```python
from build123d import *

# Parameters (mm, degrees)
F0_R     = 132.5
F0_R_2   = 9.5
F1_DEPTH = 18
F2_R     = 2
F3_R     = 132.5
F3_R_2   = 9.5
F3_R_3   = 103
F4_DEPTH = 2
F5_R     = 1.99999
F6_R     = 77.5
F7_DEPTH = 18.001
F6_R_2   = 92.6
F8_DEPTH = 11
F9_SIZE  = 3


# Not quite as in the source:
# - a fillet or chamfer is up to 0.001 mm smaller than in the source, because OpenCascade refuses the exact size


with BuildPart() as f1:
    # F0 (on Front) → F1 (new body)
    with BuildSketch(Plane.XZ):
        Circle(F0_R)
        with Locations((-44.008594722, -106.2461462388)):
            Circle(F0_R_2, mode=Mode.SUBTRACT)
        with Locations((-106.2461462388, -44.008594722)):
            Circle(F0_R_2, mode=Mode.SUBTRACT)
        with Locations((44.008594722, -106.2461462388)):
            Circle(F0_R_2, mode=Mode.SUBTRACT)
        with Locations((106.2461462388, -44.008594722)):
            Circle(F0_R_2, mode=Mode.SUBTRACT)
        with Locations((-106.2461462388, 44.008594722)):
            Circle(F0_R_2, mode=Mode.SUBTRACT)
        with Locations((-44.008594722, 106.2461462388)):
            Circle(F0_R_2, mode=Mode.SUBTRACT)
        with Locations((106.2461462388, 44.008594722)):
            Circle(F0_R_2, mode=Mode.SUBTRACT)
        with Locations((44.008594722, 106.2461462388)):
            Circle(F0_R_2, mode=Mode.SUBTRACT)
    extrude(amount=F1_DEPTH)

    # F2
    f2_edges = [f1.edges().sort_by_distance(p)[0] for p in [
        (-132.5, -18, 0),
    ]]
    fillet(f2_edges, radius=F2_R)

    # F3 (on face) → F4 (cut)
    with BuildSketch(Plane(origin=(0, 0, 0), x_dir=(-1, 0, 0), z_dir=(0, 1, 0))):
        Circle(F3_R)
        with Locations((-44.008594722, -106.2461462388)):
            Circle(F3_R_2, mode=Mode.SUBTRACT)
        with Locations((-106.2461462388, -44.008594722)):
            Circle(F3_R_2, mode=Mode.SUBTRACT)
        with Locations((44.008594722, -106.2461462388)):
            Circle(F3_R_2, mode=Mode.SUBTRACT)
        with Locations((106.2461462388, -44.008594722)):
            Circle(F3_R_2, mode=Mode.SUBTRACT)
        with Locations((-106.2461462388, 44.008594722)):
            Circle(F3_R_2, mode=Mode.SUBTRACT)
        with Locations((-44.008594722, 106.2461462388)):
            Circle(F3_R_2, mode=Mode.SUBTRACT)
        Circle(F3_R_3, mode=Mode.SUBTRACT)
        with Locations((106.2461462388, 44.008594722)):
            Circle(F3_R_2, mode=Mode.SUBTRACT)
        with Locations((44.008594722, 106.2461462388)):
            Circle(F3_R_2, mode=Mode.SUBTRACT)
    extrude(amount=-F4_DEPTH, mode=Mode.SUBTRACT)

    # F5 (radius 2 in the source; OpenCascade refuses exactly that, so slightly less here)
    f5_edges = [f1.edges().sort_by_distance(p)[0] for p in [
        (103, -2, 0),
    ]]
    fillet(f5_edges, radius=F5_R)

    # F6 (on face) → F7 (cut, through all)
    with BuildSketch(Plane(origin=(0, 0, 0), x_dir=(-1, 0, 0), z_dir=(0, 1, 0))):
        Circle(F6_R)
    extrude(amount=-F7_DEPTH, mode=Mode.SUBTRACT)

    # F6 (on face) → F8 (cut)
    with BuildSketch(Plane(origin=(0, 0, 0), x_dir=(-1, 0, 0), z_dir=(0, 1, 0))):
        Circle(F6_R_2)
        Circle(F6_R, mode=Mode.SUBTRACT)
    extrude(amount=-F8_DEPTH, mode=Mode.SUBTRACT)

    # F9
    f9_edges = [f1.edges().sort_by_distance(p)[0] for p in [
        (77.5, -18, 0),
    ]]
    chamfer(f9_edges, length=F9_SIZE)


solid = f1.part
```
Can you work these out from the model? Positions are in its coordinate system, mm. A direction names the side the tool comes from. Coordinates: 2 decimals unless noted, no trailing zeros. Return JSON: item names as keys, results as strings.
Q1. Please list where these lines run through material, in increasing order: L1, parallel to Z at x = 0, y = -13; L2, parallel to X at y = -13.75, z = 102.5; L3, parallel to Z at x = -113, y = -15.25. Write a range as from..to.
Computed values:
{"L1": "z = -132.5..-77.5, 77.5..132.5", "L2": "x = -83.96..-52.74, -35.28..35.28, 52.74..83.96", "L3": "z = -69.19..-50.69, -37.33..37.33, 50.69..69.19"}
Q2. If we section it at C-C (y = -7.75): Count the separate pieces of the cut face and the enclosed holes in it, then the cut area to 3 significant figures.
Computed values:
{"separate pieces": "1", "enclosed holes": "9", "area": "25,900 mm2"}
Q3. Thinking about a two-plate mould opening in X: for faces 1 (the cylindrical face through (-34.95, -9.89, -103.39)), 2 (the cylindrical face through (71.231, -8.902, 111.725)), 3 (the flat face through (10, -2, -107)), which applies, +X half, -X half, draft (parallel to the pull), parting line (faces both ways), or undercut?
Computed values:
{"face 1": "undercut", "face 2": "parting line", "face 3": "draft"}
Q4. On a 3-axis mill with a long thin cutter (end or side, diameter ignored), from which of +Z, -Z, +X, -X, +Y, -Y can I reach the whole of each face in a straight line? I mean faces 4 (the cylindrical face through (92.51, -5.42, 4.07)), 5 (the cylindrical face through (16.8, -12.972, -75.657)). Say none if no direction works.
Computed values:
{"face 4": "+Y", "face 5": "+Y, -Y"}
Q5. I'm going to push flat-ended pins straight in: pin 1 Ø4 at (x, y) = (-17, -12.5) entering from -Z; pin 2 Ø22 at (x, z) = (-44.01, 106.25) entering from +Y; pin 3 Ø10 at (y, z) = (-10.5, -62) entering from -X; pin 4 Ø24.5 at (x, z) = (106.25, -44.01) entering from +Y. Where does each tip first touch, or does it pass through?
Computed values:
{"pin 1": "stops at z = -131.65", "pin 2": "stops at y = -1.73", "pin 3": "stops at x = -119.61", "pin 4": "stops at y = 0"}
